For this review, take the finished solid that the model builds, in its own axes (mm). Round coordinates to 2 decimals unless told otherwise and drop trailing zeros. Loops run counter-clockwise (first coordinate to the right, second up) from the corner with the lowest first, then second, coordinate; pieces in that order, holes last. Notation, with made-up numbers: M 75,82.5 L 129,82.5 A16 cw 129,100.5 Z; hole C 9.5,73 d6. An arc over 180 degrees is marked long. Write item = value, one per line. Start each with the question number.
```python
from build123d import *

# Parameters (mm, degrees)
BOSS_EXTRUDE1_DEPTH     = 52
SKETCH2_R               = 2
CUT_EXTRUDE1_DEPTH      = 105.576527003
ESQUISSE1_R             = 2
ENL_V_MAT_EXTRU_1_DEPTH = 105.576527003
ESQUISSE2_R             = 2
ENL_V_MAT_EXTRU_2_DEPTH = 105.576527003


with BuildPart() as part:
    # Sketch1 → Boss-Extrude1 (new body)
    with BuildSketch(Plane.XY):
        with BuildLine():
            Line((0, -12.151530772), (0, 0))
            Line((0, 0), (-11.5, 0))
            Line((-11.5, 0), (-11.5, -45))
            Line((-11.5, -45), (0, -45))
            Line((0, -45), (0, -26.848469228))
            ThreePointArc((0, -26.848469228), (-6, -19.5), (0, -12.151530772))
        make_face()
        with BuildLine():
            Line((0, -45), (-11.5, -45))
            Line((-11.5, -45), (-11.5, -90))
            Line((-11.5, -90), (0, -90))
            Line((0, -90), (0, -77.848469228))
            ThreePointArc((0, -77.848469228), (-6, -70.5), (0, -63.151530772))
            Line((0, -63.151530772), (0, -45))
        make_face()
    extrude(amount=BOSS_EXTRUDE1_DEPTH)

    # Sketch2 → Cut-Extrude1 (cut, through all)
    with BuildSketch(Plane(origin=(0, 0, 0), x_dir=(0, 0, -1), z_dir=(1, 0, 0))):
        with Locations(Location((-40, -2.5, 0), (0, 0, 90))):
            Circle(SKETCH2_R)
        with Locations(Location((-40, -85, 0), (0, 0, 90))):
            Circle(SKETCH2_R)
        with Locations(Location((-12, -85, 0), (0, 0, 90))):
            Circle(SKETCH2_R)
        with Locations(Location((-12, -2.5, 0), (0, 0, 90))):
            Circle(SKETCH2_R)
    extrude(amount=-CUT_EXTRUDE1_DEPTH, mode=Mode.SUBTRACT)

    # Esquisse1 → Enlèv. mat.-Extru.1 (cut, through all)
    with BuildSketch(Plane(origin=(0, 0, 0), x_dir=(0, 0, -1), z_dir=(1, 0, 0))):
        with Locations(Location((-12, -58.25, 0), (0, 0, 90))):
            Circle(ESQUISSE1_R)
        with Locations(Location((-40, -58.25, 0), (0, 0, 90))):
            Circle(ESQUISSE1_R)
    extrude(amount=-ENL_V_MAT_EXTRU_1_DEPTH, mode=Mode.SUBTRACT)

    # Esquisse2 → Enlèv. mat.-Extru.2 (cut, through all)
    with BuildSketch(Plane(origin=(0, 0, 0), x_dir=(0, 0, -1), z_dir=(1, 0, 0))):
        with Locations(Location((-6, -39.5, 0), (0, 0, 90))):
            Circle(ESQUISSE2_R)
        with Locations(Location((-46, -39.5, 0), (0, 0, 90))):
            Circle(ESQUISSE2_R)
    extrude(amount=-ENL_V_MAT_EXTRU_2_DEPTH, mode=Mode.SUBTRACT)


solid = part.part
```
(1) Add section D-D on z = 40. Write out the cut boundary in (x, y).
(2) Add section C-C on x = -3.5. Count the separate pieces of the cut face and the enclosed holes in it, and give its area (3 significant figures).
(3) Draft analysis for pull direction Y (two halves, no side actions). For faces 1 (the cylindrical face through (-5.67, -41.498, 6.088)), 2 (the cylindrical face through (-5.67, -57.327, 38.226)), 3 (the flat face through (-6, 0, 26)), 4 (the flat face through (-7, -44, 0)), state which applies: +Y half, -Y half, draft (parallel to the pull), parting line (faces both ways), or undercut.
(4) Add section A-A on y = -58.25. Write out the cut boundary in (x, z).
(5) For pin 1 Ø2 at (x, y) = (-4.5, -71.5) entering from -Z; pin 2 Ø1.5 at (y, z) = (-49, 11) entering from +X; pin 3 Ø6 at (y, z) = (-22.5, 8) entering from +X, all flat-tipped, find the tip position at first contact; note any pin that passes through.
(6) Add section B-B on z = 6. Write out the cut boundary in (x, y).
(7) Wall thickness on L1, parallel to Z at x = -6, y = -2.5; L2, parallel to Z at x = -9, y = -39.5; L3, parallel to Y at x = -2.25, z = 2: over which ranges is each line inside the solid? List them lowest first.
Answer sheet:
q1.outline = M -11.5,-90 L 0,-90 L 0,-87 L -11.5,-87 Z; M -11.5,-83 L 0,-83 L 0,-77.85 A7.5 cw 0,-63.15 L 0,-60.25 L -11.5,-60.25 Z; M -11.5,-56.25 L 0,-56.25 L 0,-26.85 A7.5 cw 0,-12.15 L 0,-4.5 L -11.5,-4.5 Z; M -11.5,-0.5 L 0,-0.5 L 0,0 L -11.5,0 Z
q2.separate_pieces = 3
q2.enclosed_holes = 8
q2.area = 3,420 mm²
q3.face_1 = undercut
q3.face_2 = undercut
q3.face_3 = +Y half
q3.face_4 = draft
q4.outline = M -11.5,0 L 0,0 L 0,10 L -11.5,10 Z; M -11.5,14 L 0,14 L 0,38 L -11.5,38 Z; M -11.5,42 L 0,42 L 0,52 L -11.5,52 Z
q5.pin_1 = through
q5.pin_2 = 0
q5.pin_3 = -3
q6.outline = M -11.5,-90 L 0,-90 L 0,-77.85 A7.5 cw 0,-63.15 L 0,-41.5 L -11.5,-41.5 Z; M -11.5,-37.5 L 0,-37.5 L 0,-26.85 A7.5 cw 0,-12.15 L 0,0 L -11.5,0 Z
q7.L1 = 0 to 10, 14 to 38, 42 to 52
q7.L2 = 0 to 4, 8 to 44, 48 to 52
q7.L3 = -90 to -77, -64 to -26, -13 to 0
